Input: part model. Units: mm. Frame: model coordinates. A direction names the side the tool comes from. Round coordinates to 2 decimals unless told otherwise and drop trailing zeros. Order: outer loops, then holes, each group sorted by start corner. A loop starts at its lowest first (then second) coordinate and runs counter-clockwise, first axis right, second up. Notation, with made-up numbers: (1, -28) -> (27, -28) arc R19 cw to (27, -13) -> close; hole circle Ø2 at (72, -40). An arc over 180 degrees is marked (long way). Use a Markdown table: item, result.
from build123d import *

# Parameters (mm, degrees)
SKETCH1_W           = 119.2
SKETCH1_H           = 65.04
BOSS_EXTRUDE1_DEPTH = 2
SKETCH2_W           = 59.6
SKETCH2_H           = 2.5
SKETCH2_W_2         = 80
SKETCH2_H_2         = 2
BOSS_EXTRUDE2_DEPTH = 10
FILLET1_R           = 1
SKETCH4_W           = 80
SKETCH4_H           = 2.5
SKETCH4_W_2         = 8
BOSS_EXTRUDE3_DEPTH = 10
FILLET2_R           = 1
FILLET3_R           = 1
CUT_EXTRUDE2_DEPTH  = 10
CUT_EXTRUDE3_DEPTH  = 10


with BuildPart() as part:
    # Sketch1 → Boss-Extrude1 (new body)
    with BuildSketch(Plane(origin=(0, 0, 0), x_dir=(1, 0, 0), z_dir=(0, 1, 0))):
        Rectangle(SKETCH1_W, SKETCH1_H)
    extrude(amount=BOSS_EXTRUDE1_DEPTH)

    # Sketch2 → Boss-Extrude2 (add)
    with BuildSketch(Plane(origin=(0, 2, 0), x_dir=(1, 0, 0), z_dir=(0, 1, 0))):
        with Locations((0, 28.27)):
            Rectangle(SKETCH2_W, SKETCH2_H)
        with Locations((0, -5.48)):
            Rectangle(SKETCH2_W_2, SKETCH2_H_2)
    extrude(amount=BOSS_EXTRUDE2_DEPTH)

    # Fillet1
    fillet1_edges = [part.edges().sort_by_distance(p)[0] for p in [
        (40, 2, 5.48),
        (0, 2, 4.48),
        (-40, 2, 5.48),
        (-29.8, 2, -28.27),
        (29.8, 2, -28.27),
        (0, 2, -29.52),
    ]]
    fillet(fillet1_edges, radius=FILLET1_R)

    # Sketch4 → Boss-Extrude3 (add)
    with BuildSketch(Plane(origin=(0, 2, 0), x_dir=(1, 0, 0), z_dir=(0, 1, 0))):
        with Locations((0, -28.77)):
            Rectangle(SKETCH4_W, SKETCH4_H)
        with Locations((52.6, -26.27)):
            Rectangle(SKETCH4_W_2, SKETCH4_H)
    boss_extrude3 = extrude(amount=BOSS_EXTRUDE3_DEPTH)

    # Fillet2
    fillet2_edges = [part.edges().sort_by_distance(p)[0] for p in [
        (-40, 2, 28.77),
        (48.6, 2, 26.27),
        (52.6, 2, 25.02),
        (40, 2, 28.77),
        (0, 2, 27.52),
    ]]
    fillet(fillet2_edges, radius=FILLET2_R)

    # Mirror1: Boss-Extrude3 across plane
    add(boss_extrude3.mirror(Plane.ZY))

    # Fillet3
    fillet3_edges = [part.edges().sort_by_distance(p)[0] for p in [
        (-48.6, 2, 26.27),
        (-52.6, 2, 25.02),
    ]]
    fillet(fillet3_edges, radius=FILLET3_R)

    # Sketch5 → Cut-Extrude2 (cut)
    with BuildSketch(Plane(origin=(0, 2, 0), x_dir=(1, 0, 0), z_dir=(0, 1, 0))):
        with BuildLine():
            Line((46.6, 22.52), (6.311514948, 22.52))
            Line((6.311514948, 22.52), (-46.6, 22.52))
            ThreePointArc((-46.6, 22.52), (-48.721320344, 21.641320344), (-49.6, 19.52))
            Line((-49.6, 19.52), (-49.6, 3.52))
            ThreePointArc((-49.6, 3.52), (-48.721320344, 1.398679656), (-46.6, 0.52))
            Line((-46.6, 0.52), (46.6, 0.52))
            ThreePointArc((46.6, 0.52), (48.721320344, 1.398679656), (49.6, 3.52))
            Line((49.6, 3.52), (49.6, 19.52))
            ThreePointArc((49.6, 19.52), (48.721320344, 21.641320344), (46.6, 22.52))
        make_face()
    extrude(amount=-CUT_EXTRUDE2_DEPTH, mode=Mode.SUBTRACT)

    # Sketch6 → Cut-Extrude3 (cut)
    with BuildSketch(Plane(origin=(0, 2, 0), x_dir=(1, 0, 0), z_dir=(0, 1, 0))):
        with BuildLine():
            Line((54.014213562, -5.94084617), (52.045315698, -3.971948306))
            ThreePointArc((52.045315698, -3.971948306), (51.396469, -3.538402803), (50.631102135, -3.386161868))
            Line((50.631102135, -3.386161868), (46.32782558, -3.386161868))
            ThreePointArc((46.32782558, -3.386161868), (44.913612017, -3.971948306), (44.32782558, -5.386161868))
            Line((44.32782558, -5.386161868), (44.32782558, -20.397912268))
            ThreePointArc((44.32782558, -20.397912268), (44.913612017, -21.812125831), (46.32782558, -22.397912268))
            Line((46.32782558, -22.397912268), (52.6, -22.397912268))
            ThreePointArc((52.6, -22.397912268), (54.014213562, -21.812125831), (54.6, -20.397912268))
            Line((54.6, -20.397912268), (54.6, -7.355059733))
            ThreePointArc((54.6, -7.355059733), (54.447759065, -6.589692868), (54.014213562, -5.94084617))
        make_face()
        with BuildLine():
            Line((39.82782558, -13.44932419), (24.210760832, -13.44932419))
            ThreePointArc((24.210760832, -13.44932419), (23.503654051, -13.742217409), (23.210760832, -14.44932419))
            Line((23.210760832, -14.44932419), (23.210760832, -23.393622011))
            ThreePointArc((23.210760832, -23.393622011), (23.650100661, -24.454282183), (24.710760832, -24.893622011))
            Line((24.710760832, -24.893622011), (39.32782558, -24.893622011))
            ThreePointArc((39.32782558, -24.893622011), (40.388485752, -24.454282183), (40.82782558, -23.393622011))
            Line((40.82782558, -23.393622011), (40.82782558, -14.44932419))
            ThreePointArc((40.82782558, -14.44932419), (40.534932361, -13.742217409), (39.82782558, -13.44932419))
        make_face()
        with BuildLine():
            Line((4.043952302, -24.893622011), (19.660852384, -24.893622011))
            ThreePointArc((19.660852384, -24.893622011), (20.367959165, -24.600728792), (20.660852384, -23.893622011))
            Line((20.660852384, -23.893622011), (20.660852384, -14.321364431))
            ThreePointArc((20.660852384, -14.321364431), (20.221512556, -13.260704259), (19.160852384, -12.821364431))
            Line((19.160852384, -12.821364431), (4.543952302, -12.821364431))
            ThreePointArc((4.543952302, -12.821364431), (3.48329213, -13.260704259), (3.043952302, -14.321364431))
            Line((3.043952302, -14.321364431), (3.043952302, -23.893622011))
            ThreePointArc((3.043952302, -23.893622011), (3.336845521, -24.600728792), (4.043952302, -24.893622011))
        make_face()
        with BuildLine():
            Line((-4.043952302, -24.893622011), (-19.660852384, -24.893622011))
            ThreePointArc((-19.660852384, -24.893622011), (-20.367959165, -24.600728792), (-20.660852384, -23.893622011))
            Line((-20.660852384, -23.893622011), (-20.660852384, -14.321364431))
            ThreePointArc((-20.660852384, -14.321364431), (-20.221512556, -13.260704259), (-19.160852384, -12.821364431))
            Line((-19.160852384, -12.821364431), (-4.543952302, -12.821364431))
            ThreePointArc((-4.543952302, -12.821364431), (-3.48329213, -13.260704259), (-3.043952302, -14.321364431))
            Line((-3.043952302, -14.321364431), (-3.043952302, -23.893622011))
            ThreePointArc((-3.043952302, -23.893622011), (-3.336845521, -24.600728792), (-4.043952302, -24.893622011))
        make_face()
        with BuildLine():
            Line((-39.32782558, -24.893622011), (-24.710760832, -24.893622011))
            ThreePointArc((-24.710760832, -24.893622011), (-23.650100661, -24.454282183), (-23.210760832, -23.393622011))
            Line((-23.210760832, -23.393622011), (-23.210760832, -14.44932419))
            ThreePointArc((-23.210760832, -14.44932419), (-23.503654051, -13.742217409), (-24.210760832, -13.44932419))
            Line((-24.210760832, -13.44932419), (-39.82782558, -13.44932419))
            ThreePointArc((-39.82782558, -13.44932419), (-40.534932361, -13.742217409), (-40.82782558, -14.44932419))
            Line((-40.82782558, -14.44932419), (-40.82782558, -23.393622011))
            ThreePointArc((-40.82782558, -23.393622011), (-40.388485752, -24.454282183), (-39.32782558, -24.893622011))
        make_face()
        with BuildLine():
            Line((-44.32782558, -5.386161868), (-44.32782558, -20.397912268))
            ThreePointArc((-44.32782558, -20.397912268), (-44.913612017, -21.812125831), (-46.32782558, -22.397912268))
            Line((-46.32782558, -22.397912268), (-52.6, -22.397912268))
            ThreePointArc((-52.6, -22.397912268), (-54.014213562, -21.812125831), (-54.6, -20.397912268))
            Line((-54.6, -20.397912268), (-54.6, -7.355059733))
            ThreePointArc((-54.6, -7.355059733), (-54.447759065, -6.589692868), (-54.014213562, -5.94084617))
            Line((-54.014213562, -5.94084617), (-52.045315698, -3.971948306))
            ThreePointArc((-52.045315698, -3.971948306), (-51.396469, -3.538402803), (-50.631102135, -3.386161868))
            Line((-50.631102135, -3.386161868), (-46.32782558, -3.386161868))
            ThreePointArc((-46.32782558, -3.386161868), (-44.913612017, -3.971948306), (-44.32782558, -5.386161868))
        make_face()
    extrude(amount=-CUT_EXTRUDE3_DEPTH, mode=Mode.SUBTRACT)


solid = part.part
1) Cut plane B-B on x = 17.5. Return loops of the section in (y, z).
Results found:
| item | result |
|---|---|
| outline | (0, -32.52) -> (2, -32.52) -> (2, -30.52) arc R1 cw to (3, -29.52) -> (12, -29.52) -> (12, -27.02) -> (2, -27.02) -> (2, -22.52) -> (0, -22.52) -> close; (0, -0.52) -> (2, -0.52) -> (2, 3.48) arc R1 cw to (3, 4.48) -> (12, 4.48) -> (12, 6.48) -> (2, 6.48) -> (2, 12.82) -> (0, 12.82) -> close; (0, 24.89) -> (2, 24.89) -> (2, 26.52) arc R1 cw to (3, 27.52) -> (12, 27.52) -> (12, 30.02) -> (2, 30.02) -> (2, 32.52) -> (0, 32.52) -> close |
2) Cut plane C-C on z = 16. Return loops of the section in (x, y).
Results found:
| item | result |
|---|---|
| outline | (-59.6, 0) -> (-54.6, 0) -> (-54.6, 2) -> (-59.6, 2) -> close; (-44.33, 0) -> (-40.83, 0) -> (-40.83, 2) -> (-44.33, 2) -> close; (-23.21, 0) -> (-20.66, 0) -> (-20.66, 2) -> (-23.21, 2) -> close; (-3.04, 0) -> (3.04, 0) -> (3.04, 2) -> (-3.04, 2) -> close; (20.66, 0) -> (23.21, 0) -> (23.21, 2) -> (20.66, 2) -> close; (40.83, 0) -> (44.33, 0) -> (44.33, 2) -> (40.83, 2) -> close; (54.6, 0) -> (59.6, 0) -> (59.6, 2) -> (54.6, 2) -> close |
3) Cut plane A-A on z = 8.5. Return loops of the section in (x, y).
Results found:
| item | result |
|---|---|
| outline | (-59.6, 0) -> (-54.6, 0) -> (-54.6, 2) -> (-59.6, 2) -> close; (-44.33, 0) -> (44.33, 0) -> (44.33, 2) -> (-44.33, 2) -> close; (54.6, 0) -> (59.6, 0) -> (59.6, 2) -> (54.6, 2) -> close |
4) Cut plane D-D on y = 7.25. Return loops of the section in (x, z).
Results found:
| item | result |
|---|---|
| outline | (-56.6, 25.02) -> (-48.6, 25.02) -> (-48.6, 27.52) -> (-56.6, 27.52) -> close; (-40, 4.48) -> (40, 4.48) -> (40, 6.48) -> (-40, 6.48) -> close; (-40, 27.52) -> (40, 27.52) -> (40, 30.02) -> (-40, 30.02) -> close; (-29.8, -29.52) -> (29.8, -29.52) -> (29.8, -27.02) -> (-29.8, -27.02) -> close; (48.6, 25.02) -> (56.6, 25.02) -> (56.6, 27.52) -> (48.6, 27.52) -> close |
5) Set-up query: faces 4 (the flat face through (53, 7, 25.02)), 5 (the flat face through (29.8, 7, -28)), 6 (the flat face through (-52, 7, 27.52)), 7 (the flat face through (-48.6, 7, 26)). Return all of +Z, -Z, +X, -X, +Y, -Y with unobstructed straight access to the full face (end or side cutting, diameter ignored); none if empty.
Results found:
| item | result |
|---|---|
| face 4 | -Z, +X, -X, +Y |
| face 5 | -Z, +X, +Y |
| face 6 | +Z, -X, +Y |
| face 7 | +Z, -Z, +Y |
6) Pull-direction query (X, two-part tool) for faces 1 (the flat face through (48.6, 7, 26)), 2 (the flat face through (56.6, 7, 26)), 3 (the flat face through (-53, 12, 26)); classes: +X half, -X half, draft (parallel to the pull), parting line (faces both ways), or undercut.
Results found:
| item | result |
|---|---|
| face 1 | undercut |
| face 2 | +X half |
| face 3 | draft |
7) Line query: L1, parallel to Z at x = 17, y = 5; L2, parallel to Z at x = 49, y = 1; L3, parallel to Y at x = 39.5, z = 0. Output: solid intervals per line, ascending. Write a range as [from, to].
Results found:
| item | result |
|---|---|
| L1 | z = [-29.52, -27.02], [4.48, 6.48], [27.52, 30.02] |
| L2 | z = [-32.52, -21.32], [-1.72, 3.39], [22.4, 32.52] |
| L3 | y = [0, 2] |
8) Pin query (flat end, axial travel): pin 1 Ø2 at (y, z) = (7.5, 26.5) entering from +X; pin 2 Ø2 at (y, z) = (6.5, 29) entering from -X; pin 3 Ø1.2 at (y, z) = (9, 29) entering from +X; pin 4 Ø4 at (x, z) = (36.5, 5) entering from -Y. Return the tip coordinate at first contact, or that it passes through.
Results found:
| item | result |
|---|---|
| pin 1 | stops at x = 56.6 |
| pin 2 | stops at x = -40 |
| pin 3 | stops at x = 40 |
| pin 4 | stops at y = 0 |
